The listing builds one solid part. Answer for the finished solid, in the listing's coordinates (mm). Round coordinates to 2 decimals unless told otherwise and drop trailing zeros. Loops run counter-clockwise (first coordinate to the right, second up) from the corner with the lowest first, then second, coordinate; pieces in that order, holes last. Notation, with made-up numbers: (71, -5) -> (108, -5) arc R27 cw to (108, 32) -> close; hole circle Ø9 at (-18, -33.75). An arc over 180 degrees is marked (long way). Use a Markdown table: item, result. Add a question column.
Q1. Section B-B on y = 472 is taken. Give the vertices of the cut face in (x, z), then the cut area to 3 significant figures.
Q2. Consider line 1 (Y direction, x = 0, z = -13.8); line 2 (Z direction, x = -1.5, y = 621.5); line 3 (Z direction, x = 0, y = 807). Determine where each line is inside the solid, lowest interval first.
Q3. Given pin 1 Ø8 at (x, y) = (5.5, 955.5) entering from +Z; pin 2 Ø6 at (x, y) = (10.5, 946) entering from +Z; pin 3 Ø3 at (y, z) = (778, 5.5) entering from -X; pin 4 Ø6 at (x, y) = (0, 38.1) entering from -Z, each flat-ended and moving along its own axis, determine where each tip first touches the part or whether it passes through.
Q4. Section A-A on z = 0 is taken. Give the vertices of the cut face in (x, y), then the cut area to 3 significant figures.
Q5. For a pull along Z with two mould halves and no side action, classify faces 1 (the cylindrical face through (-3.62, 563.499, 16.303)), 2 (the flat face through (-1, 1143, 14)), 3 (the cylindrical face through (12.707, 563.499, 4.002)) as released by +Z, released by -Z, zero draft, split by the parting line, or undercut.
from build123d import *

# Parameters (mm, degrees)
SKETCH1_R               = 16.7005
BOSS_EXTRUDE1_DEPTH     = 1143
SKETCH2_R               = 3.429
CUT_EXTRUDE1_DEPTH      = 25.4
CUT_EXTRUDE1_DEPTH_BACK = 25.4
SKETCH3_R               = 13.3223
CUT_EXTRUDE2_DEPTH      = 1144.0000001


with BuildPart() as part:
    # Sketch1 → Boss-Extrude1 (new body)
    with BuildSketch(Plane(origin=(0, 0, 0), x_dir=(1, 0, 0), z_dir=(0, 1, 0))):
        Circle(SKETCH1_R)
    extrude(amount=BOSS_EXTRUDE1_DEPTH)

    # Sketch2 → Cut-Extrude1 (cut, two sides)
    with BuildSketch(Plane.XY) as cut_extrude1_sk:
        with Locations((0, 38.1)):
            Circle(SKETCH2_R)
        with Locations((0, 1104.9)):
            Circle(SKETCH2_R)
    extrude(amount=CUT_EXTRUDE1_DEPTH, mode=Mode.SUBTRACT)
    extrude(cut_extrude1_sk.sketch, amount=-CUT_EXTRUDE1_DEPTH_BACK, mode=Mode.SUBTRACT)

    # Sketch3 → Cut-Extrude2 (cut, through all)
    with BuildSketch(Plane.XZ):
        Circle(SKETCH3_R)
    extrude(amount=-CUT_EXTRUDE2_DEPTH, mode=Mode.SUBTRACT)


solid = part.part
Checked values:
| question | item | result |
|---|---|---|
| 1 | outline | circle Ø33.4 at (0, 0); hole circle Ø26.64 at (0, 0) |
| 1 | area | 319 mm2 |
| 2 | line 1 | y = 0 to 34.67, 41.53 to 1101.47, 1108.33 to 1143 |
| 2 | line 2 | z = -16.63 to -13.24, 13.24 to 16.63 |
| 2 | line 3 | z = -16.7 to -13.32, 13.32 to 16.7 |
| 3 | pin 1 | stops at z = 16.63 |
| 3 | pin 2 | stops at z = 14.92 |
| 3 | pin 3 | stops at x = -16.21 |
| 3 | pin 4 | passes through |
| 4 | outline | (-16.7, 0) -> (-13.32, 0) -> (-13.32, 1143) -> (-16.7, 1143) -> close; (13.32, 0) -> (16.7, 0) -> (16.7, 1143) -> (13.32, 1143) -> close |
| 4 | area | 7,720 mm2 |
| 5 | face 1 | split by the parting line |
| 5 | face 2 | zero draft |
| 5 | face 3 | undercut |
